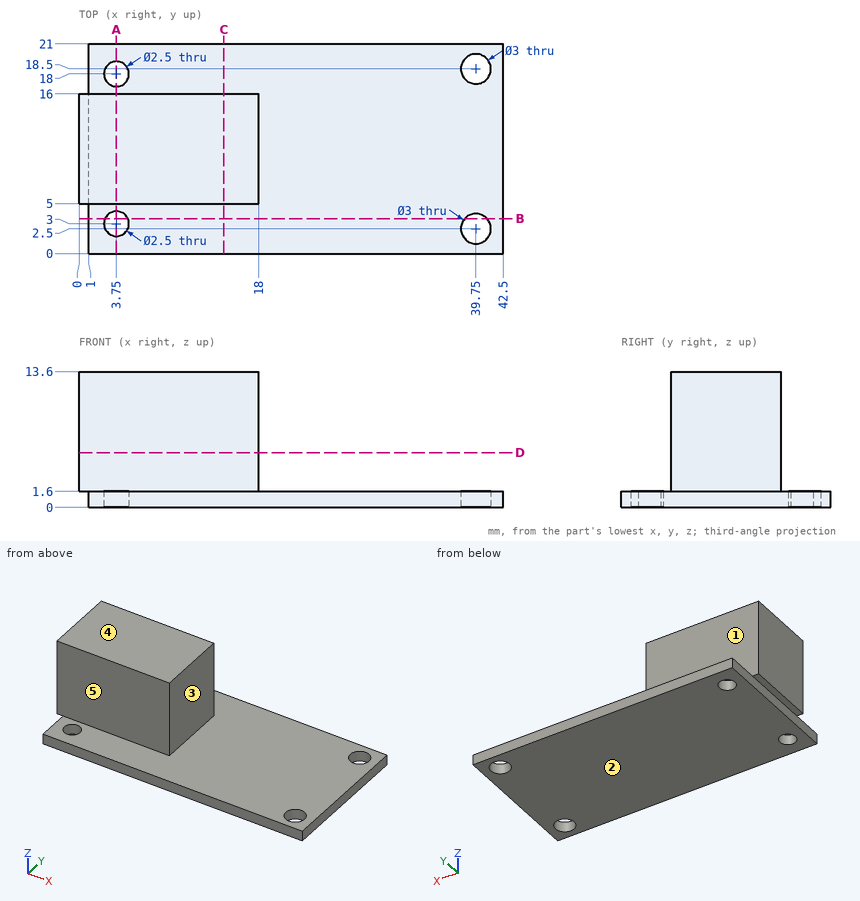
Source: three-view drawing plus pictorial views. Frame: mm from the lowest corner of the part. A direction names the side the tool comes from. Give positions to 0.01 mm unless a question says otherwise; leave off trailing zeros. Loops run counter-clockwise (first coordinate to the right, second up) from the corner with the lowest first, then second, coordinate; pieces in that order, holes last.
1) Contact query for flat-ended pins moving along their axis: pin 1 (4 mm diameter, centred on x = 8.5, z = 7.5, fed in from -Y); pin 2 (0.8 mm diameter, centred on x = 0.5, y = 12.5, fed in from -Z); pin 3 (4 mm diameter, centred on x = 39.75, y = 18.5, fed in from +Z). Output: stop coordinate, or through.
A:
pin 1: stops at y = 5
pin 2: stops at z = 1.6
pin 3: stops at z = 1.6
2) Section query B-B on y = 3.5. Return the cut outline in (x, z).
A:
outline: (1, 0) - (2.6, 0) - (2.6, 1.6) - (1, 1.6) - close; (4.9, 0) - (38.63, 0) - (38.63, 1.6) - (4.9, 1.6) - close; (40.87, 0) - (42.5, 0) - (42.5, 1.6) - (40.87, 1.6) - close
3) Reachability of the marked faces 1, 2, 3, 4 and 5 from +Z, -Z, +X, -X, +Y, -Y: full face, straight path, thin tool, end or side. Return the list, or none.
A:
face 1: +Z, +X, -X, +Y
face 2: -Z, +X, -X, +Y, -Y
face 3: +Z, +X, +Y, -Y
face 4: +Z, +X, -X, +Y, -Y
face 5: +Z, +X, -X, -Y
4) Section query C-C on x = 14.5. Return the cut outline in (y, z), and give its area (3 significant figures).
A:
outline: (0, 0) - (21, 0) - (21, 1.6) - (16, 1.6) - (16, 13.6) - (5, 13.6) - (5, 1.6) - (0, 1.6) - close
area: 166 mm2
5) Section query A-A on x = 3.75. Return the cut outline in (y, z).
A:
outline: (0, 0) - (1.75, 0) - (1.75, 1.6) - (0, 1.6) - close; (4.25, 0) - (16.75, 0) - (16.75, 1.6) - (16, 1.6) - (16, 13.6) - (5, 13.6) - (5, 1.6) - (4.25, 1.6) - close; (19.25, 0) - (21, 0) - (21, 1.6) - (19.25, 1.6) - close
6) Line query: L1, parallel to Y at x = 39.75, z = 1.15; L2, parallel to Y at x = 3.75, z = 0.9; L3, parallel to X at y = 2.5, z = 1. Output: solid intervals per line, ascending.
A:
L1: y = 0 to 1, 4 to 17, 20 to 21
L2: y = 0 to 1.75, 4.25 to 16.75, 19.25 to 21
L3: x = 1 to 2.6, 4.9 to 38.25, 41.25 to 42.5
7) Section query D-D on z = 5.5. Return the cut outline in (x, y).
A:
outline: (0, 5) - (18, 5) - (18, 16) - (0, 16) - close
